Model file for the job. Use its own axes, mm. Coordinates: 2 decimals unless noted, no trailing zeros. Order: outer loops, then holes, each group sorted by start corner. A loop starts at its lowest first (then second) coordinate and runs counter-clockwise, first axis right, second up. Notation, with made-up numbers: M 32,-13.5 L 76,-13.5 A27 ccw 76,20.5 Z; hole C 25,82.5 d9. An arc over 180 degrees is marked long. Return JSON: item names as keys, results as strings.
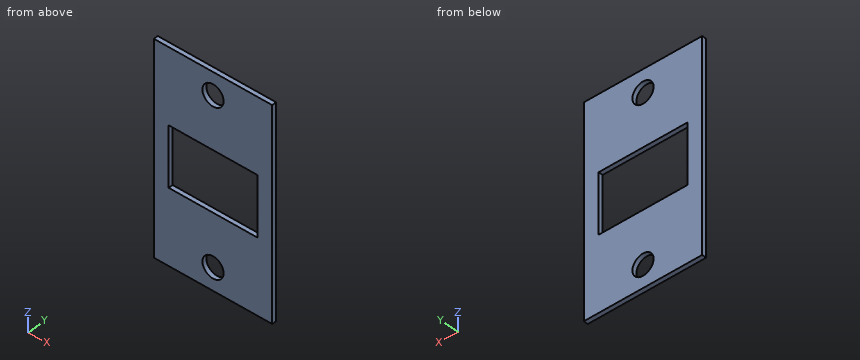
Autodesk Inventor part; units mm, degrees
ref_plane "YZ Plane" through (0, 0, 0) normal (1, 0, 0) x (0, 1, 0)
ref_plane "XZ Plane" through (0, 0, 0) normal (0, 1, 0) x (-1, 0, 0)
ref_plane "XY Plane" through (0, 0, 0) normal (0, 0, 1) x (1, 0, 0)
sketch "スケッチ1" plane through (0, 0, 0) normal (0, 1, 0) x (-1, 0, 0)
  line L0 (7.3003, 15.1278) -> (-72.6997, 15.1278)
  line L1 (-72.6997, 15.1278) -> (-72.6997, -124.8722)
  line L2 (-72.6997, -124.8722) -> (7.3003, -124.8722)
  line L3 (7.3003, -124.8722) -> (7.3003, 15.1278)
  point P0 (0, 0)
  dimension "d0" = 80
  dimension "d1" = 140
extrude "押し出し1" add sketch "スケッチ1" along normal blind 3
sketch "スケッチ2" plane through (0, 3, 0) normal (0, 1, 0) x (1, 0, 0)
  line L0 (2.6997, 34.8722) -> (62.6997, 34.8722)
  line L1 (62.6997, 34.8722) -> (62.6997, 74.8722)
  line L2 (62.6997, 74.8722) -> (2.6997, 74.8722)
  line L3 (2.6997, 74.8722) -> (2.6997, 34.8722)
  circle A0 centre (32.6997, -0.1278) radius 7.15
  circle A1 centre (32.6997, 109.8722) radius 7.15
  line L4 (-7.3003, -15.1278) -> (72.6997, -15.1278)
  line L5 (72.6997, 124.8722) -> (-7.3003, 124.8722)
  line L6 (-7.3003, 124.8722) -> (-7.3003, -15.1278)
  point P0 (0, 0)
  dimension "d4" = 60
  dimension "d5" = 40
  dimension "d6" = 14.3
  dimension "d7" = 14.3
  dimension "d8" = 15
  dimension "d9" = 15
  dimension "d10" = 40
  dimension "d11" = 40
  dimension "d12" = 10
  dimension "d13" = 50
extrude "押し出し2" cut sketch "スケッチ2" against normal blind 3
equation "\"BendRadius\" = Thickness"
equation "\"BendReliefWidth\" = Thickness"
equation "\"BendReliefDepth\" = 0.5 * Thickness"
equation "\"CornerReliefSize\" = 4 * Thickness"
equation "\"MinimumRemnant\" = 2 * Thickness"
equation "\"TransitionRadius\" = BendRadius"
equation "\"JacobiRadiusSize\" = BendRadius"
equation "\"GapSize\" = Thickness"
properties part number "came2"
Item 1: Saw through at D-D (y = 2.2). Write the cut outline in (x, z), and give its area (3 significant figures).
Check result:
{"outline": "M -7.3,-124.87 L 72.7,-124.87 L 72.7,15.13 L -7.3,15.13 Z; hole M 2.7,-74.87 L 62.7,-74.87 L 62.7,-34.87 L 2.7,-34.87 Z; hole C 32.7,-109.87 d14.3; hole C 32.7,0.13 d14.3", "area": "8,480 mm2"}
Item 2: Wall check: line 1 (Z direction, x = 8, y = 1.8); line 2 (X direction, y = 0.4, z = -62); line 3 (Z direction, x = 33.5, y = 2.55). Give the ranges that are in metal, low to high.
Check result:
{"line 1": "z = -124.87 to -74.87, -34.87 to 15.13", "line 2": "x = -7.3 to 2.7, 62.7 to 72.7", "line 3": "z = -124.87 to -116.98, -102.77 to -74.87, -34.87 to -6.98, 7.23 to 15.13"}
Item 3: Saw through at B-B (z = -59.5). Write the cut outline in (x, y), and give its area (3 significant figures).
Check result:
{"outline": "M -7.3,0 L 2.7,0 L 2.7,3 L -7.3,3 Z; M 62.7,0 L 72.7,0 L 72.7,3 L 62.7,3 Z", "area": "60.0 mm2"}
Item 4: Saw through at C-C (x = 30.5). Write the cut outline in (y, z), and give its area (3 significant figures).
Check result:
{"outline": "M 0,-124.87 L 3,-124.87 L 3,-116.68 L 0,-116.68 Z; M 0,-103.07 L 3,-103.07 L 3,-74.87 L 0,-74.87 Z; M 0,-34.87 L 3,-34.87 L 3,-6.68 L 0,-6.68 Z; M 0,6.93 L 3,6.93 L 3,15.13 L 0,15.13 Z", "area": "218 mm2"}
Item 5: Saw through at A-A (x = 58.5). Write the cut outline in (y, z), and give its area (3 significant figures).
Check result:
{"outline": "M 0,-124.87 L 3,-124.87 L 3,-74.87 L 0,-74.87 Z; M 0,-34.87 L 3,-34.87 L 3,15.13 L 0,15.13 Z", "area": "300 mm2"}
